For this review, take the finished solid that the model builds, in its own axes (mm). A direction names the side the tool comes from. Round coordinates to 2 decimals unless told otherwise and drop trailing zeros. Order: outer loops, then holes, each group sorted by start corner. A loop starts at its lowest first (then second) coordinate and runs counter-clockwise, first axis right, second up.
from build123d import *

# Parameters (mm, degrees)
CHAMFER_1_SIZE = 1


with BuildPart() as part:
    # Эскиз1 → Повернуть1 (revolve)
    with BuildSketch(Plane.XY, mode=Mode.PRIVATE) as revolve_1_sk:
        Polygon((-5.5, 10), (5.5, 10), (5.5, 12), (12.5, 12), (12.5, 15.5), (4.9, 15.5), (4.9, 25), (-4.9, 25), (-4.9, 15.5), (-12.5, 15.5), (-12.5, 12), (-5.5, 12), align=None)
    revolve(revolve_1_sk.sketch.rotate(Axis((-24.618848289, 0, 0), (1, 0, 0)), 90), axis=Axis((-24.618848289, 0, 0), (1, 0, 0)))  # turned: the seam where the file's is

    # Фаска1
    chamfer_1_edges = [part.edges().sort_by_distance(p)[0] for p in [
        (-4.9, 0, -25),
        (4.9, 0, -25),
    ]]
    chamfer(chamfer_1_edges, length=CHAMFER_1_SIZE)


solid = part.part
(1) Add section A-A on z = 0. Give the boundary of the cut face in (x, y).
(2) Draft analysis for pull direction Z (two halves, no side actions). For faces 1 (the face through (-8.951, -3.604, 11.446)), 2 (the face through (-8.753, -15.368, -2.018)), 3 (the face through (12.5, 11.4, -4.5)), state which applies: pulls with the +Z half, pulls with the -Z half, needs draft (parallel to the pull), parting line crosses it, or undercut.
(3) Add section D-D on x = 2.75. Give the boundary of the cut face in (y, z), plus the area to 3 significant figures.
(4) Tool access review of faces 4 (the face through (-5.5, -9, -5)), 5 (the face through (0, 0, -10)), 6 (the face through (5.5, -9, 5)): name each direction out of +Z, -Z, +X, -X, +Y, -Y from which nothing blocks a thin tool from reaching the whole face with its end or side.
(5) Add section C-C on x = -8.5. Give the boundary of the cut face in (y, z).
(6) Clearance check with flat-ended pins moving along their axes: P1, Ø1.5, axis at x = 5.5, z = 16.5, coming from the +Y side; P2, Ø7, axis at y = -4, z = 4.5, coming from the +X side; P3, Ø1.5, axis at y = 17, z = -9, coming from the +X side; P4, Ø21.5, axis at y = 0, z = 0, coming from the -X side. State where each tip first meets the part, or that it passes through.
(7) Wall thickness on L1, parallel to Y at x = -8.75, z = 0; L2, parallel to X at y = -18, z = 5.5; L3, parallel to Y at x = 1.5, z = 0: over which ranges is each line inside the solid? List them lowest first.
Here are the results:
1. outline: (-12.5, -15.5) - (-4.9, -15.5) - (-4.9, -24) - (-3.9, -25) - (3.9, -25) - (4.9, -24) - (4.9, -15.5) - (12.5, -15.5) - (12.5, -12) - (5.5, -12) - (5.5, -10) - (-5.5, -10) - (-5.5, -12) - (-12.5, -12) - close; (-12.5, 12) - (-5.5, 12) - (-5.5, 10) - (5.5, 10) - (5.5, 12) - (12.5, 12) - (12.5, 15.5) - (4.9, 15.5) - (4.9, 24) - (3.9, 25) - (-3.9, 25) - (-4.9, 24) - (-4.9, 15.5) - (-12.5, 15.5) - close
2. face 1: undercut
2. face 2: parting line crosses it
2. face 3: needs draft
3. outline: circle Ø50 at (0, 0); hole circle Ø20 at (0, 0)
3. area: 1,650 mm2
4. face 4: -X
4. face 5: +X, -X
4. face 6: +X
5. outline: circle Ø31 at (0, 0); hole circle Ø24 at (0, 0)
6. P1: stops at y = 17.85
6. P2: passes through
6. P3: stops at x = 4.9
6. P4: stops at x = -5.5
7. L1: y = -15.5 to -12, 12 to 15.5
7. L2: x = -4.9 to 4.9
7. L3: y = -25 to -10, 10 to 25
